from build123d import *

# Parameters (mm, degrees)
F0_W      = 40.2
F0_H      = 40
F1_DEPTH  = 5.5
F2_R      = 2.85
F3_DEPTH  = 3.5
F4_R      = 1.6
F5_DEPTH  = 25
F6_W      = 4.8
F6_H      = 40
F7_DEPTH  = 2
F8_SIZE   = 1.8
F9_R      = 1.6
F10_DEPTH = 25
F11_R     = 2.85
F12_DEPTH = 3.5


with BuildPart() as f1:
    # F0 (on Top) → F1 (new body)
    with BuildSketch(Plane.XY):
        with Locations((20.1, 20)):
            Rectangle(F0_W, F0_H)
    extrude(amount=F1_DEPTH)

    # F2 (on face) → F3 (cut)
    with BuildSketch(Plane.XY.offset(5.5)):
        with Locations((35.2, 6.5)):
            Circle(F2_R)
        with Locations((35.2, 33.5)):
            Circle(F2_R)
        with Locations((5, 33.5)):
            Circle(F2_R)
        with Locations((5, 6.5)):
            Circle(F2_R)
    extrude(amount=-F3_DEPTH, mode=Mode.SUBTRACT)

    # F4 (on face) → F5 (cut)
    with BuildSketch(Plane.XY.offset(5.5)):
        with Locations((35.2, 33.5)):
            Circle(F4_R)
        with Locations((35.2, 6.5)):
            Circle(F4_R)
        with Locations((5, 33.5)):
            Circle(F4_R)
        with Locations((5, 6.5)):
            Circle(F4_R)
    extrude(amount=-F5_DEPTH, mode=Mode.SUBTRACT)

    # F6 (on face) → F7 (join)
    with BuildSketch(Plane(origin=(0, 0, 0), x_dir=(1, 0, 0), z_dir=(0, 0, -1))):
        with Locations((20.1, -20)):
            Rectangle(F6_W, F6_H)
    extrude(amount=F7_DEPTH)

    # F8
    f8_edges = [f1.edges().sort_by_distance(p)[0] for p in [
        (17.7, 20, -2),
        (22.5, 20, -2),
    ]]
    chamfer(f8_edges, length=F8_SIZE)

    # F9 (on face) → F10 (cut)
    with BuildSketch(Plane(origin=(0, 0, -2), x_dir=(1, 0, 0), z_dir=(0, 0, -1))):
        with Locations((20.1, -30)):
            Circle(F9_R)
        with Locations((20.1, -10)):
            Circle(F9_R)
    extrude(amount=-F10_DEPTH, mode=Mode.SUBTRACT)

    # F11 (on face) → F12 (cut)
    with BuildSketch(Plane.XY.offset(5.5)):
        with Locations((20.1, 30)):
            Circle(F11_R)
        with Locations((20.1, 10)):
            Circle(F11_R)
    extrude(amount=-F12_DEPTH, mode=Mode.SUBTRACT)


solid = f1.part
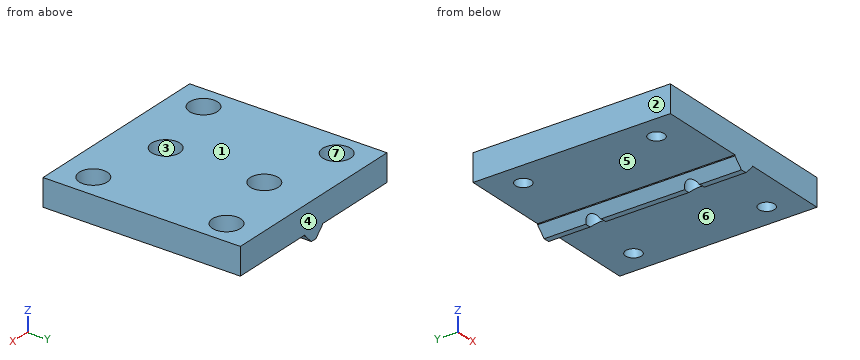
Work out the finished part from the listing and answer in its coordinate system (mm). Face numbers are marked on the shaded views. A direction names the side the tool comes from. Round coordinates to 2 decimals unless told otherwise and drop trailing zeros. Loops run counter-clockwise (first coordinate to the right, second up) from the corner with the lowest first, then second, coordinate; pieces in that order, holes last. Notation, with made-up numbers: (-6.75, -7) - (37.25, -7) arc R32 ccw to (37.25, 25) - close; hole circle Ø1 at (7.25, 23.5). An arc over 180 degrees is marked (long way). Use one line per item in the form item = value. Start each with the question number.
(1) Consider line 1 (Y direction, x = 35.2, z = 2.9); line 2 (Y direction, x = 20.1, z = 0.95); line 3 (X direction, y = 36, z = 4). Determine where each line is inside the solid, lowest interval first.
(2) Determine the mould class of the marked faces 1, 2 and 3 for opening direction X: +X half, -X half, draft (parallel to the pull), parting line (faces both ways), or undercut.
(3) Find section C-C on z = 3.25. Determine the outline of the cut face in (x, y).
(4) Flat-ended cylindrical pins translate along their axes: P1, Ø1.7, axis at x = 19, y = 31.5, coming from the +Z side; P2, Ø6.5, axis at x = 21, y = 9, coming from the +Z side; P3, Ø14, axis at x = 31.5, y = 19.5, coming from the -Z side. Find the tip coordinate at first contact, or state that the pin passes through.
(5) Which of the six approach directions +Z, -Z, +X, -X, +Y, -Y give full straight-line access (tool end or side, diameter ignored) to the marked faces 4, 5, 6 and 7?
(6) Find section B-B on x = 5. Determine the outline of the cut face in (y, z), and give its area (3 significant figures).
(7) Find section D-D on y = 33.5. Determine the outline of the cut face in (x, z), and give its area (3 significant figures).
(8) Find section A-A on y = 10. Determine the outline of the cut face in (x, z).
Answer list:
q1.line_1 = 0 to 3.65, 9.35 to 30.65, 36.35 to 40
q1.line_2 = 0 to 8.4, 11.6 to 28.4, 31.6 to 40
q1.line_3 = 0 to 3.63, 6.37 to 33.83, 36.57 to 40.2
q2.face_1 = draft
q2.face_2 = -X half
q2.face_3 = undercut
q3.outline = (0, 0) - (40.2, 0) - (40.2, 40) - (0, 40) - close; hole circle Ø5.7 at (5, 6.5); hole circle Ø5.7 at (5, 33.5); hole circle Ø5.7 at (20.1, 10); hole circle Ø5.7 at (20.1, 30); hole circle Ø5.7 at (35.2, 6.5); hole circle Ø5.7 at (35.2, 33.5)
q4.P1 = 2
q4.P2 = 5.5
q4.P3 = 0
q5.face_4 = +Z, -Z, +X, -X, +Y
q5.face_5 = -Z, -X, +Y, -Y
q5.face_6 = -Z, +X, +Y, -Y
q5.face_7 = +Z
q6.outline = (0, 0) - (4.9, 0) - (4.9, 2) - (3.65, 2) - (3.65, 5.5) - (0, 5.5) - close; (8.1, 0) - (31.9, 0) - (31.9, 2) - (30.65, 2) - (30.65, 5.5) - (9.35, 5.5) - (9.35, 2) - (8.1, 2) - close; (35.1, 0) - (40, 0) - (40, 5.5) - (36.35, 5.5) - (36.35, 2) - (35.1, 2) - close
q6.area = 167 mm^2
q7.outline = (0, 0) - (3.4, 0) - (3.4, 2) - (2.15, 2) - (2.15, 5.5) - (0, 5.5) - close; (6.6, 0) - (17.7, 0) - (17.7, -0.2) - (19.5, -2) - (20.7, -2) - (22.5, -0.2) - (22.5, 0) - (33.6, 0) - (33.6, 2) - (32.35, 2) - (32.35, 5.5) - (7.85, 5.5) - (7.85, 2) - (6.6, 2) - close; (36.8, 0) - (40.2, 0) - (40.2, 5.5) - (38.05, 5.5) - (38.05, 2) - (36.8, 2) - close
q7.area = 175 mm^2
q8.outline = (0, 0) - (17.7, 0) - (17.7, -0.2) - (18.5, -1) - (18.5, 2) - (17.25, 2) - (17.25, 5.5) - (0, 5.5) - close; (21.7, -1) - (22.5, -0.2) - (22.5, 0) - (40.2, 0) - (40.2, 5.5) - (22.95, 5.5) - (22.95, 2) - (21.7, 2) - close
